Read the model definition and answer for the solid it produces. Units are mm, in the model's axes. Face numbers are marked on the shaded views. A direction names the side the tool comes from. Round coordinates to 2 decimals unless told otherwise and drop trailing zeros. Order: outer loops, then holes, each group sorted by start corner. A loop starts at its lowest first (then second) coordinate and runs counter-clockwise, first axis right, second up. Notation, with made-up numbers: (83.5, 63.25) -> (88.5, 63.25) arc R34 cw to (88.5, 94.25) -> close; hole circle Ø5 at (-24.5, -34.75). An arc over 180 degrees is marked (long way). Answer as a JSON object with one key per item and string values. Group by question number.
Item 1: For the marked faces 1 and 2, determine the directions among +Z, -Z, +X, -X, +Y, -Y from which every point of the face is accessible in a straight line to the end or side of a thin tool.
Item 2: The mould has two halves that part along Z. Classify the marked faces 3 and 4: pulls with the +Z half, pulls with the -Z half, needs draft (parallel to the pull), parting line crosses it, or undercut.
Item 3: Section C-C, the plane x = -46 is taken. Write down the section's boundary in (y, z), plus the area to 3 significant figures.
Item 4: Section B-B, the plane y = 12.5 is taken. Write down the section's boundary in (x, z), plus the area to 3 significant figures.
Item 5: Section D-D, the plane z = 27 is taken. Write down the section's boundary in (x, y).
Item 6: Given P1, Ø6, axis at x = 32.5, y = 31.5, coming from the -Z side; P2, Ø8, axis at y = 15.5, z = 40, coming from the -X side; P3, Ø8, axis at y = 43.5, z = 54.5, coming from the -X side, each flat-ended and moving along its own axis, determine where each tip first touches the part or whether it passes through.
Item 7: Section A-A, the plane z = 97 is taken. Write down the section's boundary in (x, y), plus the area to 3 significant figures.
Item 8: Consider probe 1 along Y at (x, z) = (9, 65); probe 2 along X at (y, z) = (5.5, 89.5); probe 3 along Y at (x, z) = (18, 92). Determine where each line is inside the solid, lowest interval first. Write a range as from..to.
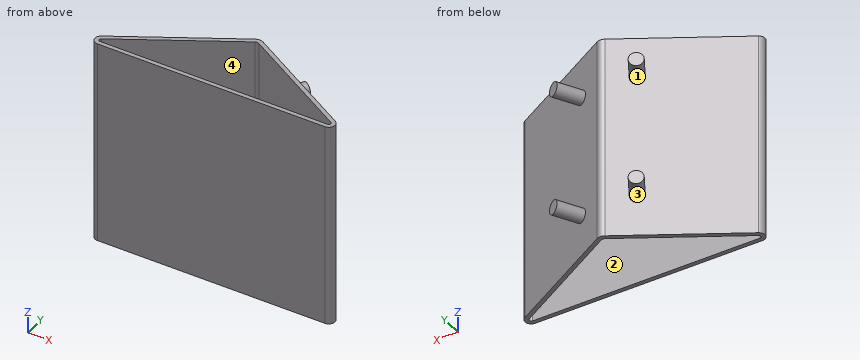
from build123d import *

# Parameters (mm, degrees)
F1_DEPTH = 150
F2_R     = 5
F3_DEPTH = 20


# Not quite as in the source:
# - a pattern or mirror of a feature is missing from the dataset's text; its kind, count and spacing are read off the source's solid


with BuildPart() as f1:
    # F0 (on Top) → F1 (new body)
    with BuildSketch(Plane.XY):
        with BuildLine():
            Line((-83.2057713659, 0), (0, 0))
            Line((0, 0), (83.2057713659, 0))
            ThreePointArc((83.2057713659, 0), (87.5524375842, 3.335314297), (85.4557713659, 8.397114317))
            Line((85.4557713659, 8.397114317), (3, 56.0029761114))
            ThreePointArc((3, 56.0029761114), (0, 56.8068236887), (-3, 56.0029761114))
            Line((-3, 56.0029761114), (-85.4557713659, 8.397114317))
            ThreePointArc((-85.4557713659, 8.397114317), (-87.5524375842, 3.335314297), (-83.2057713659, 0))
        make_face()
        with BuildLine():
            Line((83.2057713659, 3), (0, 3))
            Line((0, 3), (-83.2057713659, 3))
            ThreePointArc((-83.2057713659, 3), (-84.6546601054, 4.1117714323), (-83.9557713659, 5.7990381057))
            Line((-83.9557713659, 5.7990381057), (-1.5, 53.4048999))
            ThreePointArc((-1.5, 53.4048999), (0, 53.8068236887), (1.5, 53.4048999))
            Line((1.5, 53.4048999), (83.9557713659, 5.7990381057))
            ThreePointArc((83.9557713659, 5.7990381057), (84.6546601054, 4.1117714323), (83.2057713659, 3))
        make_face(mode=Mode.SUBTRACT)
    extrude(amount=F1_DEPTH)

    # F2 (on face) → F3 (join)
    with BuildSketch(Plane(origin=(-25, 43.3012701892, 0), x_dir=(-0.8660254038, -0.5, 0), z_dir=(-0.5, 0.8660254038, 0))):
        with Locations((-5.4034118443, 30)):
            Circle(F2_R)
        with Locations((-5.4034118443, 120)):
            Circle(F2_R)
    f3 = extrude(amount=F3_DEPTH)

    # F3_copies: F3 across plane
    add(f3.mirror(Plane(origin=(0, 0, 0), x_dir=(0, 0, 1), z_dir=(1, 0, 0))))


solid = f1.part
Values found:
{
 "1": {"face 1": "none", "face 2": "+Z, -Z"},
 "2": {"face 3": "undercut", "face 4": "needs draft"},
 "3": {"outline": "(0, 0) -> (3, 0) -> (3, 150) -> (0, 150) -> close; (27.71, 0) -> (31.18, 0) -> (31.18, 150) -> (27.71, 150) -> close", "area": "970 mm2"},
 "4": {"outline": "(-78.35, 0) -> (-72.35, 0) -> (-72.35, 150) -> (-78.35, 150) -> close; (72.35, 0) -> (78.35, 0) -> (78.35, 150) -> (72.35, 150) -> close", "area": "1,800 mm2"},
 "5": {"outline": "(-85.46, 8.4) arc R4.5 ccw to (-83.21, 0) -> (83.21, 0) arc R4.5 ccw to (85.46, 8.4) -> (23.78, 44) -> (33.78, 61.32) -> (26.86, 65.32) -> (16.86, 48) -> (3, 56) arc R6 ccw to (-3, 56) -> (-16.86, 48) -> (-26.86, 65.32) -> (-33.78, 61.32) -> (-23.78, 44) -> close; hole (-83.96, 5.8) arc R1.5 ccw to (-83.21, 3) -> (83.21, 3) arc R1.5 ccw to (83.96, 5.8) -> (1.5, 53.4) arc R3 ccw to (-1.5, 53.4) -> close"},
 "6": {"P1": "through", "P2": "x = -80.08", "P3": "x = -31.58"},
 "7": {"outline": "(-85.46, 8.4) arc R4.5 ccw to (-83.21, 0) -> (83.21, 0) arc R4.5 ccw to (85.46, 8.4) -> (3, 56) arc R6 ccw to (-3, 56) -> close; hole (-83.96, 5.8) arc R1.5 ccw to (-83.21, 3) -> (83.21, 3) arc R1.5 ccw to (83.96, 5.8) -> (1.5, 53.4) arc R3 ccw to (-1.5, 53.4) -> close", "area": "1,130 mm2"},
 "8": {"probe 1": "0..3, 49.07..52.54", "probe 2": "-87.59..-84.32, 84.32..87.59", "probe 3": "0..3, 43.88..47.34"}
}
